Here's how the part is built. I have some questions about the finished solid (model axes, mm). Face numbers are marked on the shaded views. A direction names the side the tool comes from. Coordinates: 2 decimals unless noted, no trailing zeros. Write each loop counter-clockwise with the first axis right and the second up, starting at its lowest first coordinate (ties: lowest second). Pieces come first, ordered by that corner, then holes. Notation, with made-up numbers: (83, 80.5) -> (135, 80.5) arc R12 cw to (135, 90.5) -> close; hole circle Ø11 at (54, 34). An arc over 180 degrees is marked (long way). Put each result on its own line as item: value. Start each with the question number.
Item 1: On a 3-axis mill with a long thin cutter (end or side, diameter ignored), from which of +Z, -Z, +X, -X, +Y, -Y can I reach the whole of each face in a straight line? I mean the marked faces 4 and 5. Say none if no direction works.
Item 2: I want a section at D-D, the plane y = -5.25. List the corners of the cut face in (x, z) for me.
Item 3: If we mould it in two halves opening along X, with no side actions, what happens to the marked faces 1, 2 and 3? For each: released by +X, released by -X, zero draft, split by the parting line, or undercut.
Item 4: For pin 1 (1.5 mm diameter, centred on y = -1, z = -0.5, fed in from +X); pin 2 (3 mm diameter, centred on x = -1.5, y = -4, fed in from +Z), each with a flat end and sliding along its axis, tell me the tip position at first contact or that it passes through.
Item 5: I need wall thicknesses on line 1 (Z direction, x = 0, y = -0.25); line 2 (Y direction, x = -1.25, z = 1.25); line 3 (Z direction, x = -0.75, y = -2.25). Which ranges of each line are inside material? Lowest first, please. Write a range as [from, to].
Item 6: I want a section at C-C, the plane y = -3.25. List the corners of the cut face in (x, z) for me.
Item 7: I want a section at B-B, the plane z = 0. List the corners of the cut face in (x, y) for me.
Item 8: I want a section at A-A, the plane x = 0. List the corners of the cut face in (y, z) for me.
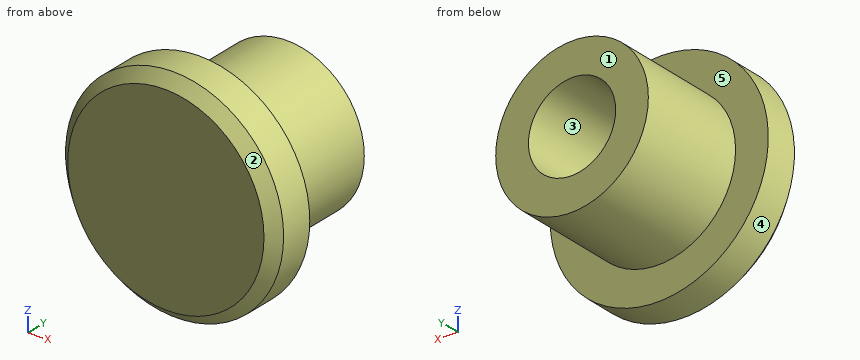
from build123d import *

# Parameters (mm, degrees)
F0_R     = 3.5
F1_DEPTH = 5
F2_R     = 5
F2_R_2   = 3.5
F3_DEPTH = 2
F4_R     = 2
F5_DEPTH = 5
F6_SIZE  = 0.5


with BuildPart() as f1:
    # F0 (on Front) → F1 (new body)
    with BuildSketch(Plane.XZ):
        Circle(F0_R)
    extrude(amount=F1_DEPTH)

    # F2 (on face) → F3 (join)
    with BuildSketch(Plane.XZ.offset(5)):
        Circle(F2_R)
        Circle(F2_R_2, mode=Mode.SUBTRACT)
        Circle(F2_R_2)
    extrude(amount=F3_DEPTH)

    # F4 (on face) → F5 (cut, through all)
    with BuildSketch(Plane(origin=(0, 0, 0), x_dir=(-1, 0, 0), z_dir=(0, 1, 0))):
        Circle(F4_R)
    extrude(amount=-F5_DEPTH, mode=Mode.SUBTRACT)

    # F6
    f6_edges = [f1.edges().sort_by_distance(p)[0] for p in [
        (-5, -7, 0),
    ]]
    chamfer(f6_edges, length=F6_SIZE)


solid = f1.part
Calculated:
1. face 4: +Y, -Y
1. face 5: +Y
2. outline: circle Ø10 at (0, 0)
3. face 1: zero draft
3. face 2: split by the parting line
3. face 3: undercut
4. pin 1: stops at x = 3.5
4. pin 2: stops at z = 4.99
5. line 1: z = [-3.5, -2], [2, 3.5]
5. line 2: y = [-7, -5]
5. line 3: z = [-3.42, -1.85], [1.85, 3.42]
6. outline: circle Ø7 at (0, 0); hole circle Ø4 at (0, 0)
7. outline: (-5, -6.5) -> (-4.5, -7) -> (4.5, -7) -> (5, -6.5) -> (5, -5) -> (3.5, -5) -> (3.5, 0) -> (2, 0) -> (2, -5) -> (-2, -5) -> (-2, 0) -> (-3.5, 0) -> (-3.5, -5) -> (-5, -5) -> close
8. outline: (-7, -4.5) -> (-6.5, -5) -> (-5, -5) -> (-5, -3.5) -> (0, -3.5) -> (0, -2) -> (-5, -2) -> (-5, 2) -> (0, 2) -> (0, 3.5) -> (-5, 3.5) -> (-5, 5) -> (-6.5, 5) -> (-7, 4.5) -> close
